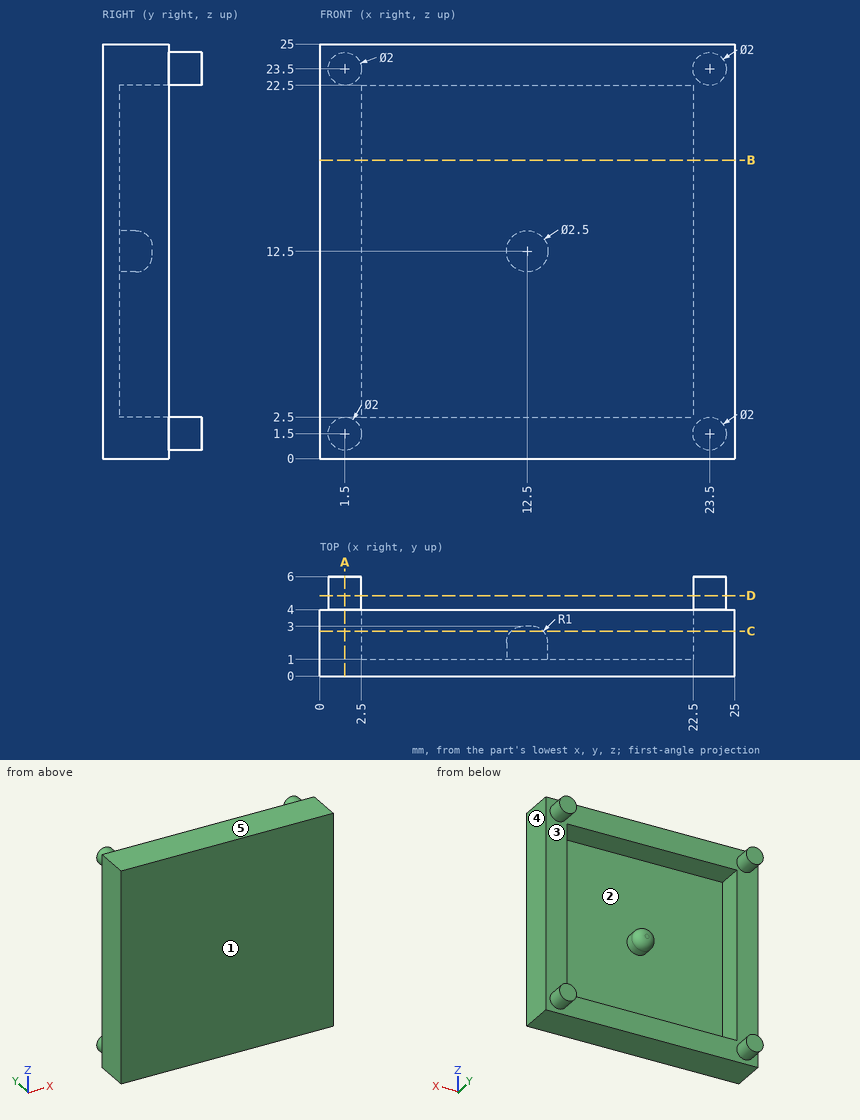
The drawing under review shows one solid part. Ordinate dimensions are in mm from its lowest x, y, z. A direction names the side the tool comes from. Coordinates: 2 decimals unless noted, no trailing zeros. Write each loop counter-clockwise with the first axis right and the second up, starting at its lowest first coordinate (ties: lowest second). Pieces come first, ordered by that corner, then holes. Notation, with made-up numbers: (-16.5, 67) - (-0.5, 67) arc R11 ccw to (-0.5, 86) - close; hole circle Ø10 at (37, -11.75). An arc over 180 degrees is marked (long way). Use one line per item in the form item = value.
Q1. The part is to be moulded in two halves that separate along X. For the marked faces 3, 4 and 5, say which applies: +X half, -X half, draft (parallel to the pull), parting line (faces both ways), or undercut.
Taken from the geometry:
face_3 = undercut
face_4 = +X half
face_5 = draft
Q2. For probe 1 along Z at (x, y) = (20, 1.95); probe 2 along Y at (x, z) = (12.5, 12.25), list the stretches that pass through material, from the lowest coordinate up.
Taken from the geometry:
probe_1 = 0 to 2.5, 22.5 to 25
probe_2 = 0 to 3
Q3. Consider section C-C (y = 2.7). Count the separate pieces of the cut face and the enclosed holes in it, plus the area to 3 significant figures.
Taken from the geometry:
separate_pieces = 2
enclosed_holes = 1
area = 228 mm^2
Q4. Machinability: for the marked faces 1 and 2, which of the approach directions +Z, -Z, +X, -X, +Y, -Y give a long, thin tool a straight path to every point of the face, cutting with its end or side? Answer none if there is none.
Taken from the geometry:
face_1 = +Z, -Z, +X, -X, -Y
face_2 = +Y
Q5. Insertion check: pin 1 Ø4 at (x, z) = (8.5, 22) entering from +Y; pin 2 Ø10 at (x, z) = (14.5, 10.5) entering from +Y; pin 3 Ø2 at (y, z) = (5.5, 20) entering from +X. Each pin has a flat end and moves straight along its axis. Give the tip position at first contact, or say it passes through.
Taken from the geometry:
pin_1 = 4
pin_2 = 3
pin_3 = through
Q6. Consider section A-A (x = 1.5). Write out the cut boundary in (y, z), plus the area to 3 significant figures.
Taken from the geometry:
outline = (0, 0) - (4, 0) - (4, 0.5) - (6, 0.5) - (6, 2.5) - (4, 2.5) - (4, 22.5) - (6, 22.5) - (6, 24.5) - (4, 24.5) - (4, 25) - (0, 25) - close
area = 108 mm^2
Q7. Consider section D-D (y = 4.85). Write out the cut boundary in (x, z).
Taken from the geometry:
outline = circle Ø2 at (1.5, 1.5); circle Ø2 at (1.5, 23.5); circle Ø2 at (23.5, 1.5); circle Ø2 at (23.5, 23.5)
Q8. Consider section B-B (z = 18). Write out the cut boundary in (x, y).
Taken from the geometry:
outline = (0, 0) - (25, 0) - (25, 4) - (22.5, 4) - (22.5, 1) - (2.5, 1) - (2.5, 4) - (0, 4) - close
